from build123d import *

# Parameters (mm, degrees)
SCHIZZO1_R                   = 3.375
ESTRUSIONE_ESTRUSIONE1_DEPTH = 4
RACCORDO1_R                  = 6
RACCORDO4_R                  = 6
RACCORDO5_R                  = 6
RACCORDO6_R                  = 6
RACCORDO8_R                  = 10
RACCORDO9_R                  = 10
RACCORDO10_R                 = 10
RACCORDO11_R                 = 10
SCHIZZO2_R                   = 0.5
TAGLIO_ESTRUSIONE1_DEPTH     = 58.835974964


with BuildPart() as part:
    # Schizzo1 → Estrusione-Estrusione1 (new body)
    with BuildSketch(Plane(origin=(0, 0, 0), x_dir=(1, 0, 0), z_dir=(0, 1, 0))):
        with BuildLine():
            ThreePointArc((0, 7.376524617), (1.042643641, 3.590434154), (2.633357109, 0))
            Line((2.633357109, 0), (49.366642891, 0))
            ThreePointArc((49.366642891, 0), (50.957356359, 3.590434154), (52, 7.376524617))
            Line((52, 7.376524617), (52, 17.623475383))
            ThreePointArc((52, 17.623475383), (50.957356359, 21.409565846), (49.366642891, 25))
            Line((49.366642891, 25), (2.633357109, 25))
            ThreePointArc((2.633357109, 25), (1.042643641, 21.409565846), (0, 17.623475383))
            Line((0, 17.623475383), (0, 7.376524617))
        make_face()
        with BuildLine():
            Line((17.5, 22), (35.1, 22))
            ThreePointArc((35.1, 22), (35.948528137, 21.648528137), (36.3, 20.8))
            Line((36.3, 20.8), (36.3, 19.2))
            ThreePointArc((36.3, 19.2), (35.948528137, 18.351471863), (35.1, 18))
            Line((35.1, 18), (17.5, 18))
            ThreePointArc((17.5, 18), (16.651471863, 18.351471863), (16.3, 19.2))
            Line((16.3, 19.2), (16.3, 20.8))
            ThreePointArc((16.3, 20.8), (16.651471863, 21.648528137), (17.5, 22))
        make_face(mode=Mode.SUBTRACT)
        with Locations(Location((25, 8.22, 0), (0, 0, 270))):
            Circle(SCHIZZO1_R, mode=Mode.SUBTRACT)
        with BuildLine():
            Line((5, 15.5), (5, 20.5))
            Line((5, 20.5), (13, 20.5))
            Line((13, 20.5), (13, 14.1))
            Line((13, 14.1), (14.5, 14.1))
            Line((14.5, 14.1), (14.5, 11.1))
            ThreePointArc((14.5, 11.1), (14.792893219, 10.392893219), (15.5, 10.1))
            Line((15.5, 10.1), (16.5, 10.1))
            Line((16.5, 10.1), (16.5, 6.1))
            Line((16.5, 6.1), (13, 6.1))
            Line((13, 6.1), (13, 4.5))
            Line((13, 4.5), (5, 4.5))
            Line((5, 4.5), (5, 9.5))
            Line((5, 9.5), (7.8, 9.5))
            ThreePointArc((7.8, 9.5), (8.507106781, 9.792893219), (8.8, 10.5))
            Line((8.8, 10.5), (8.8, 14.5))
            ThreePointArc((8.8, 14.5), (8.507106781, 15.207106781), (7.8, 15.5))
            Line((7.8, 15.5), (5, 15.5))
        make_face(mode=Mode.SUBTRACT)
        with BuildLine():
            Line((36, 10.3), (37, 10.3))
            ThreePointArc((37, 10.3), (37.707106781, 10.592893219), (38, 11.3))
            Line((38, 11.3), (38, 14.3))
            Line((38, 14.3), (39.5, 14.3))
            Line((39.5, 14.3), (39.5, 20.5))
            Line((39.5, 20.5), (47.5, 20.5))
            Line((47.5, 20.5), (47.5, 15.5))
            Line((47.5, 15.5), (44.7, 15.5))
            ThreePointArc((44.7, 15.5), (43.992893219, 15.207106781), (43.7, 14.5))
            Line((43.7, 14.5), (43.7, 10.5))
            ThreePointArc((43.7, 10.5), (43.992893219, 9.792893219), (44.7, 9.5))
            Line((44.7, 9.5), (47.5, 9.5))
            Line((47.5, 9.5), (47.5, 4.5))
            Line((47.5, 4.5), (39.5, 4.5))
            Line((39.5, 4.5), (39.5, 6.3))
            Line((39.5, 6.3), (36, 6.3))
            Line((36, 6.3), (36, 10.3))
        make_face(mode=Mode.SUBTRACT)
    extrude(amount=ESTRUSIONE_ESTRUSIONE1_DEPTH)

    # Raccordo1
    raccordo1_edges = [part.edges().sort_by_distance(p)[0] for p in [
        (2.633357109, 2, -25),
    ]]
    fillet(raccordo1_edges, radius=RACCORDO1_R)

    # Raccordo4
    raccordo4_edges = [part.edges().sort_by_distance(p)[0] for p in [
        (2.633357109, 2, 0),
    ]]
    fillet(raccordo4_edges, radius=RACCORDO4_R)

    # Raccordo5
    raccordo5_edges = [part.edges().sort_by_distance(p)[0] for p in [
        (49.366642891, 2, -25),
    ]]
    fillet(raccordo5_edges, radius=RACCORDO5_R)

    # Raccordo6
    raccordo6_edges = [part.edges().sort_by_distance(p)[0] for p in [
        (49.366642891, 2, 0),
    ]]
    fillet(raccordo6_edges, radius=RACCORDO6_R)

    # Raccordo8
    raccordo8_edges = [part.edges().sort_by_distance(p)[0] for p in [
        (0, 2, -7.376524617),
    ]]
    fillet(raccordo8_edges, radius=RACCORDO8_R)

    # Raccordo9
    raccordo9_edges = [part.edges().sort_by_distance(p)[0] for p in [
        (0, 2, -17.623475383),
    ]]
    fillet(raccordo9_edges, radius=RACCORDO9_R)

    # Raccordo10
    raccordo10_edges = [part.edges().sort_by_distance(p)[0] for p in [
        (52, 2, -17.623475383),
    ]]
    fillet(raccordo10_edges, radius=RACCORDO10_R)

    # Raccordo11
    raccordo11_edges = [part.edges().sort_by_distance(p)[0] for p in [
        (52, 2, -7.376524617),
    ]]
    fillet(raccordo11_edges, radius=RACCORDO11_R)

    # Schizzo2 → Taglio-Estrusione1 (cut, through all)
    with BuildSketch(Plane.XZ):
        with Locations(Location((25, -14.42, 0), (0, 0, 270))):
            Circle(SCHIZZO2_R)
        with Locations(Location((31.7, -8.22, 0), (0, 0, 270))):
            Circle(SCHIZZO2_R)
        with Locations(Location((18.5, -8.22, 0), (0, 0, 270))):
            Circle(SCHIZZO2_R)
        with Locations(Location((25, -2.02, 0), (0, 0, 270))):
            Circle(SCHIZZO2_R)
    extrude(amount=-TAGLIO_ESTRUSIONE1_DEPTH, mode=Mode.SUBTRACT)


solid = part.part
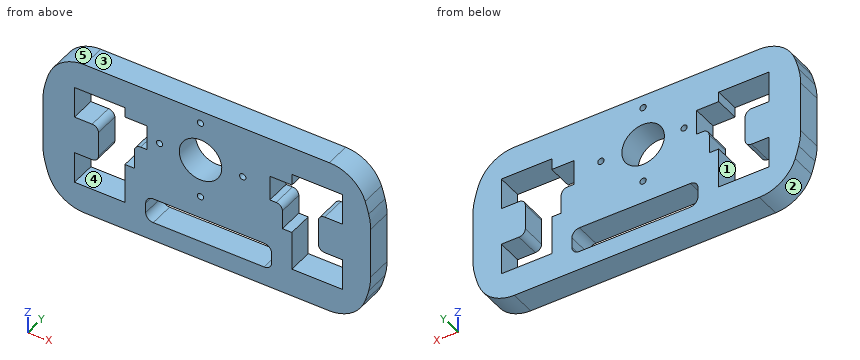
Geometry check sheet. Reference: the model listing, model coordinates, mm. Face numbers are marked on the shaded views. A direction names the side the tool comes from. Round coordinates to 2 decimals unless told otherwise and drop trailing zeros. Order: outer loops, then holes, each group sorted by start corner. A loop starts at its lowest first (then second) coordinate and runs counter-clockwise, first axis right, second up. Notation, with made-up numbers: M -4,17.25 L 43,17.25 A28 cw 43,35.25 Z; hole C -16.5,-37.75 d6. An arc over 180 degrees is marked long. Answer in a Markdown table with one row per item. Add a question column.
Item 1: Draft check along X on the marked faces 3, 4 and 5. Enter one of: released by +X, released by -X, zero draft, split by the parting line, or undercut.
Item 2: Set-up check for the marked faces 1 and 2: record each of +Z, -Z, +X, -X, +Y, -Y from which the full face is reachable in a straight line by a thin tool's end or side.
Item 3: Sectioned sample at B-B, the plane x = 18.5. Enter the section's corners in (y, z).
Item 4: Material ranges on L1, parallel to X at y = 1.85, z = -13; L2, parallel to X at y = 1.05, z = -14.42; L3, parallel to Z at x = 45.5, y = 0.4, recorded low to high. Write a range as [from, to].
Item 5: Sectioned sample at C-C, the plane x = 37.5. Enter the section's corners in (y, z), plus the area to 3 significant figures.
Item 6: Depth check by flat-ended pin: pin 1 Ø1.2 at (y, z) = (2.5, -18) entering from -X; pin 2 Ø0.8 at (y, z) = (3, -20) entering from -X; pin 3 Ø1.4 at (x, y) = (46.5, 1.5) entering from -Z. Enter the tip coordinate at first touch or a pass-through.
Item 7: Sectioned sample at D-D, the plane y = 2.4. State how many separate pieces and enclosed holes the cut face has, plus the area to 3 significant figures.
Item 8: Sectioned sample at A-A, the plane x = 25. Enter the section's corners in (y, z) (3 decimals).
Filled in:
| question | item | result |
|---|---|---|
| 1 | face 3 | zero draft |
| 1 | face 4 | undercut |
| 1 | face 5 | released by -X |
| 2 | face 1 | +Y, -Y |
| 2 | face 2 | -Z, -X, +Y, -Y |
| 3 | outline | M 0,-25 L 4,-25 L 4,-22 L 0,-22 Z; M 0,-18 L 4,-18 L 4,-8.72 L 0,-8.72 Z; M 0,-7.72 L 4,-7.72 L 4,0 L 0,0 Z |
| 4 | L1 | x = [0, 8.8], [14.5, 38], [43.7, 52] |
| 4 | L2 | x = [0, 8.8], [13, 24.5], [25.5, 39.5], [43.7, 52] |
| 4 | L3 | z = [-25, -20.5], [-15.5, -9.5], [-4.5, 0] |
| 5 | outline | M 0,-25 L 4,-25 L 4,-10.43 L 0,-10.43 Z; M 0,-6.3 L 4,-6.3 L 4,0 L 0,0 Z |
| 5 | area | 83.5 mm² |
| 6 | pin 1 | stops at x = 0.04 |
| 6 | pin 2 | stops at x = 0.47 |
| 6 | pin 3 | stops at z = -24.99 |
| 7 | separate pieces | 1 |
| 7 | enclosed holes | 8 |
| 7 | area | 886 mm² |
| 8 | outline | M 0,-25 L 4,-25 L 4,-22 L 0,-22 Z; M 0,-18 L 4,-18 L 4,-14.92 L 0,-14.92 Z; M 0,-13.92 L 4,-13.92 L 4,-11.595 L 0,-11.595 Z; M 0,-4.845 L 4,-4.845 L 4,-2.52 L 0,-2.52 Z; M 0,-1.52 L 4,-1.52 L 4,0 L 0,0 Z |
